Could you check a few things on this model? Use its own coordinates, in mm. A direction names the side the tool comes from. Round coordinates to 2 decimals unless told otherwise and drop trailing zeros. Order: outer loops, then holes, each group sorted by start corner. A loop starts at its lowest first (then second) coordinate and runs counter-clockwise, first axis right, second up.
```python
from build123d import *

# Parameters (mm, degrees)
SKETCH1_W           = 140
SKETCH1_H           = 20
BOSS_EXTRUDE1_DEPTH = 80
SKETCH2_W           = 10
SKETCH2_H           = 80
CUT_EXTRUDE1_DEPTH  = 10
SKETCH3_R           = 7.5
SKETCH3_R_2         = 5.25
CUT_EXTRUDE2_DEPTH  = 80
SKETCH4_R           = 2.5
CUT_EXTRUDE4_DEPTH  = 440


with BuildPart() as part:
    # Sketch1 → Boss-Extrude1 (new body)
    with BuildSketch(Plane.XY):
        with Locations((70, -10)):
            Rectangle(SKETCH1_W, SKETCH1_H)
    extrude(amount=BOSS_EXTRUDE1_DEPTH)

    # Sketch2 → Cut-Extrude1 (cut)
    with BuildSketch(Plane(origin=(0, 0, 0), x_dir=(1, 0, 0), z_dir=(0, 1, 0))):
        with Locations((135, -40)):
            Rectangle(SKETCH2_W, SKETCH2_H)
        with Locations((5, -40)):
            Rectangle(SKETCH2_W, SKETCH2_H)
    extrude(amount=-CUT_EXTRUDE1_DEPTH, mode=Mode.SUBTRACT)

    # Sketch3 → Cut-Extrude2 (cut)
    with BuildSketch(Plane.XY.offset(80)):
        with Locations((20, -10)):
            Circle(SKETCH3_R)
        with Locations((70, -10)):
            Circle(SKETCH3_R_2)
        with Locations((120, -10)):
            Circle(SKETCH3_R)
    extrude(amount=-CUT_EXTRUDE2_DEPTH, mode=Mode.SUBTRACT)

    # Sketch4 → Cut-Extrude4 (cut)
    with BuildSketch(Plane(origin=(0, -10, 0), x_dir=(1, 0, 0), z_dir=(0, 1, 0))):
        with Locations(Location((5.056286957, -10, 0), (0, 0, 270))):
            Circle(SKETCH4_R)
        with Locations(Location((5.056286957, -30, 0), (0, 0, 270))):
            Circle(SKETCH4_R)
        with Locations(Location((5.056286957, -50, 0), (0, 0, 270))):
            Circle(SKETCH4_R)
        with Locations(Location((5.056286957, -70, 0), (0, 0, 270))):
            Circle(SKETCH4_R)
        with Locations(Location((134.943713043, -70, 0), (0, 0, 270))):
            Circle(SKETCH4_R)
        with Locations(Location((134.943713043, -50, 0), (0, 0, 270))):
            Circle(SKETCH4_R)
        with Locations(Location((134.943713043, -30, 0), (0, 0, 270))):
            Circle(SKETCH4_R)
        with Locations(Location((134.943713043, -10, 0), (0, 0, 270))):
            Circle(SKETCH4_R)
    extrude(amount=-CUT_EXTRUDE4_DEPTH, mode=Mode.SUBTRACT)


solid = part.part
```
Q1. We'd pull the mould along Y, two halves only. Please class faces 1 (the flat face through (69, -20, 39)), 2 (the cylindrical face through (127.154, -7.747, 40.56)), 3 (the cylindrical face through (137.052, -14.93, 11.344)): released by +Y, released by -Y, zero draft, split by the parting line, or undercut.
Q2. Imagine slicing it at A-A, the plane z = 70. Please give me the cut outline in (x, y), then the cut area to 3 significant figures.
Q3. Imagine slicing it at C-C, the plane x = 20. Please give me the cut outline in (y, z), then the cut area to 3 significant figures.
Q4. For P1, Ø8, axis at x = 134.94, z = 70, coming from the -Y side; P2, Ø11, axis at x = 3.5, z = 52.5, coming from the +Y side; P3, Ø12, axis at y = -3, z = 27.5, coming from the +X side; P4, Ø5, axis at y = -6, z = 42, coming from the -X side, each with a flat end and sliding along its axis, tell me the tip position at first contact or that it passes through.
Q5. Imagine slicing it at D-D, the plane z = 35. Please give me the cut outline in (x, y), then the cut area to 3 significant figures.
Q6. I need wall thicknesses on L1, parallel to X at y = -13.25, z = 50; L2, parallel to X at y = -10.5, z = 26; L3, parallel to X at y = -3.25, z = 28. Which ranges of each line are inside material? Lowest first, please.
Q7. For faces 4 (the flat face through (69, -17, 80)), 5 (the flat face through (135, -10, 39)), 6 (the flat face through (10, -5, 41)), which set-ups out of +Z, -Z, +X, -X, +Y, -Y let a thin tool reach every point of the face, with its end or its side?
Q8. Imagine slicing it at B-B, the plane y = -12. State how many separate pieces and enclosed holes the cut face has, then the cut area to 3 significant figures.
Filled in:
1. face 1: released by -Y
1. face 2: undercut
1. face 3: zero draft
2. outline: (0, -20) - (2.56, -20) - (2.56, -10) - (0, -10) - close; (7.56, -20) - (132.44, -20) - (132.44, -10) - (130, -10) - (130, 0) - (10, 0) - (10, -10) - (7.56, -10) - close; (137.44, -20) - (140, -20) - (140, -10) - (137.44, -10) - close; hole circle Ø15 at (20, -10); hole circle Ø10.5 at (70, -10); hole circle Ø15 at (120, -10)
2. area: 2,060 mm2
3. outline: (-20, 0) - (-17.5, 0) - (-17.5, 80) - (-20, 80) - close; (-2.5, 0) - (0, 0) - (0, 80) - (-2.5, 80) - close
3. area: 400 mm2
4. P1: stops at y = -20
4. P2: stops at y = -10
4. P3: stops at x = 130
4. P4: stops at x = 10
5. outline: (0, -20) - (140, -20) - (140, -10) - (130, -10) - (130, 0) - (10, 0) - (10, -10) - (0, -10) - close; hole circle Ø15 at (20, -10); hole circle Ø10.5 at (70, -10); hole circle Ø15 at (120, -10)
5. area: 2,160 mm2
6. L1: x = 0 to 2.56, 7.56 to 13.24, 26.76 to 65.88, 74.12 to 113.24, 126.76 to 132.44, 137.44 to 140
6. L2: x = 0 to 12.52, 27.48 to 64.77, 75.23 to 112.52, 127.48 to 140
6. L3: x = 10 to 16.73, 23.27 to 116.73, 123.27 to 130
7. face 4: +Z, +X, -X, +Y, -Y
7. face 5: +Z, -Z, +X, +Y
7. face 6: +Z, -Z, -X, +Y
8. separate pieces: 4
8. enclosed holes: 8
8. area: 7,950 mm2
